Autodesk Inventor part; units mm, degrees
ref_plane "YZ Plane" through (0, 0, 0) normal (1, 0, 0) x (0, 1, 0)
ref_plane "XZ Plane" through (0, 0, 0) normal (0, 1, 0) x (-1, 0, 0)
ref_plane "XY Plane" through (0, 0, 0) normal (0, 0, 1) x (1, 0, 0)
sketch "Sketch1" plane through (0, 0, 0) normal (0, 0, 1) x (1, 0, 0)
  line L0 (-30.48, 28.575) -> (20.32, 28.575)
  line L1 (20.32, 28.575) -> (20.32, -28.575)
  line L2 (20.32, -28.575) -> (-30.48, -28.575)
  line L3 (-30.48, -28.575) -> (-30.48, 28.575)
  line L4 (-25.4, 28.575) -> (25.4, -28.575) construction
  line L5 (25.4, 28.575) -> (-25.4, -28.575) construction
  line L6 (0, 0) -> (0, -19.5531)
  dimension "d0" = 50.8
  dimension "d1" = 57.15
  dimension "d2" = 20.32
  dimension "d3" = 0
extrude "Extrusion1" add sketch "Sketch1" along normal blind 1.27
sketch "Sketch2" plane through (0, 0, 1.27) normal (0, 0, 1) x (1, 0, 0)
  line L0 (-30.48, -28.575) -> (20.32, -28.575)
  line L1 (20.32, -28.575) -> (20.32, 28.575)
  line L2 (20.32, 28.575) -> (-30.48, 28.575)
  line L3 (-30.48, 28.575) -> (-30.48, -28.575)
  line L4 (20.32, 28.575) -> (-30.48, 28.575)
  line L5 (-30.48, -28.575) -> (20.32, -28.575)
  line L6 (20.32, 28.575) -> (-30.48, 28.575)
  line L7 (-30.48, 28.575) -> (-30.48, -28.575)
  line L8 (-30.48, -28.575) -> (20.32, -28.575)
  line L9 (20.32, -28.575) -> (20.32, 28.575)
  line L10 (22.86, 31.115) -> (-30.48, 31.115)
  line L11 (-30.48, -31.115) -> (22.86, -31.115)
  line L12 (22.86, -31.115) -> (22.86, 31.115)
  line L13 (-30.48, 31.115) -> (-30.48, 28.575)
  line L14 (-30.48, 28.575) -> (-30.48, -28.575)
  line L15 (-30.48, -28.575) -> (-30.48, -31.115)
  point P0 (0, 0)
  point P1 (-30.48, 28.575)
  dimension "d6" = 2.54
  dimension "d7" = 2.54
  dimension "d8" = 2.54
extrude "Extrusion2" add sketch "Sketch2" against normal blind 63.5 contours L0 L1 L2 L13 L10 L12 L11 L15
fillet "Fillet1" radius 38.1 2 edges at (-30.48, -29.845, -62.23) (-30.48, 29.845, -62.23)
sketch "Sketch3" plane through (0, 0, 0) normal (0, 0, -1) x (-1, 0, 0)
  line L0 (30.48, -28.575) -> (-20.32, -28.575)
  line L1 (30.48, 28.575) -> (30.48, -28.575)
  line L2 (-20.32, 28.575) -> (30.48, 28.575)
  line L3 (-20.32, -28.575) -> (-20.32, 28.575)
  line L4 (-7.62, -31.115) -> (30.48, -31.115)
  line L5 (30.48, -31.115) -> (30.48, -28.575)
  line L6 (30.48, -28.575) -> (-7.62, -28.575)
  line L7 (-7.62, -28.575) -> (-7.62, -31.115)
  line L8 (30.48, 31.115) -> (-7.62, 31.115)
  line L9 (-7.62, 31.115) -> (-7.62, 28.575)
  line L10 (30.48, 28.575) -> (30.48, 28.575)
  line L11 (30.48, 28.575) -> (30.48, 31.115)
  line L12 (-20.32, 28.575) -> (30.48, 28.575)
  line L13 (30.48, 28.575) -> (30.48, 28.575)
  line L14 (30.48, -28.575) -> (-20.32, -28.575)
  line L15 (26.416, -28.575) -> (23.876, -28.575)
  line L16 (23.876, -28.575) -> (23.876, -26.035)
  line L17 (23.876, -26.035) -> (26.416, -26.035)
  line L18 (26.416, -26.035) -> (26.416, -28.575)
  line L19 (21.336, -28.575) -> (18.796, -28.575)
  line L20 (18.796, -28.575) -> (18.796, -22.225)
  line L21 (18.796, -22.225) -> (21.336, -22.225)
  line L22 (21.336, -22.225) -> (21.336, -28.575)
  line L23 (-20.32, 28.575) -> (30.48, 28.575)
  line L24 (26.416, 28.575) -> (23.876, 28.575)
  line L25 (23.876, 28.575) -> (23.876, 26.035)
  line L26 (23.876, 26.035) -> (26.416, 26.035)
  line L27 (26.416, 26.035) -> (26.416, 28.575)
  line L28 (21.336, 28.575) -> (18.796, 28.575)
  line L29 (18.796, 28.575) -> (18.796, 22.225)
  line L30 (18.796, 22.225) -> (21.336, 22.225)
  line L31 (21.336, 22.225) -> (21.336, 28.575)
  point P0 (0, 0)
  point P1 (30.48, -26.035)
  point P2 (23.876, -28.575)
  point P3 (30.48, 26.035)
  point P4 (23.876, 28.575)
  point P5 (21.336, 28.575)
  point P6 (18.796, 28.575)
  dimension "d12" = 2.54
  dimension "d13" = 2.54
  dimension "d14" = 2.54
  dimension "d15" = 6.35
  dimension "d16" = 2.54
  dimension "d17" = 2.54
  dimension "d18" = 2.54
  dimension "d19" = 2.54
  dimension "d20" = 6.35
  dimension "d21" = 2.54
  dimension "d57" = 6.35
  dimension "d58" = 6.35
  dimension "d59" = 4.064
extrude "Extrusion3" add sketch "Sketch3" along normal blind 25.4 contours L0 L16 L17 L18 | L27 L26 L25 L2 | L0 L20 L21 L22 | L31 L30 L29 L2
sketch "Sketch4" plane through (-30.48, -31.115, 1.27) normal (0, -1, 0) x (1, 0, 0)
  arc A0 (35.54, -42.8168) -> (35.14, -42.4168) centre (35.14, -42.8168) ccw
  line L0 (35.54, -42.8168) -> (35.54, -47.1668)
  line L1 (35.54, -47.1668) -> (37.14, -47.1668)
  line L2 (37.14, -47.1668) -> (37.14, -42.8168)
  arc A1 (37.54, -42.4168) -> (37.14, -42.8168) centre (37.54, -42.8168) ccw
  line L3 (37.54, -42.4168) -> (53.14, -42.4168)
  line L4 (53.14, -42.4168) -> (53.14, -20.3168)
  line L5 (53.14, -20.3168) -> (37.54, -20.3168)
  arc A2 (37.14, -19.9168) -> (37.54, -20.3168) centre (37.54, -19.9168) ccw
  line L6 (37.14, -19.9168) -> (37.14, -15.5668)
  line L7 (37.14, -15.5668) -> (35.54, -15.5668)
  line L8 (35.54, -15.5668) -> (35.54, -19.9168)
  arc A3 (35.14, -20.3168) -> (35.54, -19.9168) centre (35.14, -19.9168) ccw
  line L9 (35.14, -20.3168) -> (31.04, -20.3168)
  line L10 (31.04, -20.3168) -> (31.04, -35.0805)
  spline S0 degree 3 poles (31.04, -35.0805) (31.04, -35.2107) (31.032, -35.3398) (31.0199, -35.4684) (31.0078, -35.597) (30.9913, -35.725) (30.9724, -35.8527) (30.9346, -36.1082) (30.8875, -36.3608) (30.84, -36.6168) knots 0 0 0 0 0.00039 0.00039 0.00039 0.000781 0.000781 0.000781 0.001562 0.001562 0.001562 0.001562
  spline S1 degree 3 poles (30.84, -36.6168) (30.8871, -36.8706) (30.9346, -37.1252) (30.9724, -37.3806) (30.9913, -37.5084) (31.0077, -37.6365) (31.0199, -37.7651) (31.032, -37.8937) (31.04, -38.0228) (31.04, -38.153) knots -0.000015 -0.000015 -0.000015 -0.000015 0.000759 0.000759 0.000759 0.001147 0.001147 0.001147 0.001534 0.001534 0.001534 0.001534
  line L11 (31.04, -38.153) -> (31.04, -42.4168)
  line L12 (31.04, -42.4168) -> (35.14, -42.4168)
  line L13 (37.34, -42.8168) -> (37.34, -47.1668)
  line L14 (37.34, -15.5668) -> (37.34, -19.9168)
  line L15 (37.34, -42.8168) -> (53.34, -42.8168)
  line L16 (53.34, -42.8168) -> (53.34, -47.1668)
  line L17 (53.34, -47.1668) -> (37.34, -47.1668)
  line L18 (37.34, -47.1668) -> (37.34, -42.8168)
  line L19 (37.34, -19.9168) -> (53.34, -19.9168)
  line L20 (53.34, -19.9168) -> (53.34, -15.5668)
  line L21 (53.34, -15.5668) -> (37.34, -15.5668)
  line L22 (37.34, -15.5668) -> (37.34, -19.9168)
  line L23 (53.34, 0) -> (53.34, -63.5)
  point P0 (30.48, -1.27)
  dimension "d33" = 0
  dimension "d34" = 0
extrude "Extrusion4" add sketch "Sketch4" along normal blind 12.7 contours L15 L16 L17 L13 | L19 L14 L21 L20
sketch "Sketch5" plane through (20.32, -28.575, 0) normal (-1, 0, 0) x (0, 0, 1)
  line L0 (0, 0) -> (0, 57.15)
  line L1 (0, 57.15) -> (-62.23, 57.15)
  line L2 (-62.23, 0) -> (-62.23, 57.15)
  line L3 (0, 0) -> (-62.23, 0)
  line L4 (-62.23, 59.69) -> (-62.23, -2.54)
  line L5 (-62.23, 28.575) -> (-2.2668, 28.575)
  line L6 (-31.1958, 28.575) -> (-31.115, 57.15)
  line L7 (-31.115, 57.15) -> (-37.465, 57.15)
  line L8 (0, 57.15) -> (-62.23, 57.15)
  line L9 (-37.465, 57.15) -> (-37.465, 0)
  line L10 (-62.23, 0) -> (-24.13, 0)
  line L11 (-37.465, 32.1945) -> (-31.1958, 35.814)
  line L12 (-31.1958, 35.814) -> (-24.9267, 32.1945)
  line L13 (-24.9267, 32.1945) -> (-24.9267, 24.9555)
  line L14 (-24.9267, 24.9555) -> (-31.1958, 21.336)
  line L15 (-31.1958, 21.336) -> (-37.465, 24.9555)
  line L16 (-37.465, 24.9555) -> (-37.465, 32.1945)
  point P0 (0, 28.575)
  point P1 (-37.465, 28.575)
  point P2 (-37.465, 32.1945)
  point P3 (-37.465, 24.9555)
  dimension "d28" = 57.15
  dimension "d30" = 6.35
  dimension "d67" = 7.239
extrude "Extrusion5" cut sketch "Sketch5" against normal blind 2.54 contours L12 L13 L5 L6 | L6 L5 L9 L11 L12 | L9 L5 L13 L14 L15
sketch "Sketch6" plane through (-30.48, 31.115, 1.27) normal (0, 1, 0) x (1, 0, 0)
  circle A0 centre (29.21, 44.45) radius 2.54
  line L0 (53.34, 0) -> (53.34, 63.5)
  line L1 (53.34, 0) -> (0, 0)
  point P0 (30.48, 1.27)
  dimension "d38" = 5.08
  dimension "d41" = 24.13
  dimension "d42" = 44.45
extrude "Extrusion6" cut sketch "Sketch6" against normal blind 2.54
chamfer "Chamfer3" distance 12.7 angle 25 1 edges at (14.86, -31.115, -45.8968) measured on face at (17.5267, -39.5817, -45.8968)
chamfer "Chamfer4" distance 12.7 angle 25 1 edges at (14.86, -31.115, -14.2968) measured on face at (17.5267, -39.5817, -14.2968)
sketch "Sketch8" plane through (-30.48, -43.815, 1.27) normal (0, -1, 0) x (1, 0, 0)
  line L0 (53.34, -42.8168) -> (37.34, -42.8168)
  line L1 (50.5178, -53.0889) -> (46.99, -53.0889)
  line L2 (46.99, -53.0889) -> (46.99, -42.8168)
  line L3 (46.99, -42.8168) -> (50.5178, -42.8168)
  line L4 (50.5178, -42.8168) -> (50.5178, -53.0889)
  line L5 (37.34, -53.0889) -> (53.34, -53.0889)
  line L6 (53.34, -53.0889) -> (53.34, -47.1668)
  point P0 (30.48, -1.27)
  dimension "d52" = 2.8222
  dimension "d53" = 6.35
extrude "Extrusion7" cut sketch "Sketch8" against normal blind 12.7
sketch "Sketch9" plane through (0, 0, 0) normal (0, 0, -1) x (-1, 0, 0)
  line L0 (18.796, -22.225) -> (21.336, -22.225)
  line L1 (21.336, -22.225) -> (21.336, -28.575)
  line L2 (23.876, -28.575) -> (21.336, -28.575)
  line L3 (23.876, -28.575) -> (23.876, -26.035)
  line L4 (23.876, -26.035) -> (26.416, -26.035)
  line L5 (26.416, -26.035) -> (26.416, -28.575)
  line L6 (30.48, -28.575) -> (26.416, -28.575)
  line L7 (30.48, 28.575) -> (30.48, -28.575)
  line L8 (26.416, 28.575) -> (30.48, 28.575)
  line L9 (26.416, 28.575) -> (26.416, 26.035)
  line L10 (26.416, 26.035) -> (23.876, 26.035)
  line L11 (23.876, 26.035) -> (23.876, 28.575)
  line L12 (21.336, 28.575) -> (23.876, 28.575)
  line L13 (21.336, 28.575) -> (21.336, 22.225)
  line L14 (21.336, 22.225) -> (18.796, 22.225)
  line L15 (-20.32, 28.575) -> (18.796, 28.575)
  line L16 (-20.32, -28.575) -> (-20.32, 28.575)
  line L17 (18.796, -28.575) -> (-20.32, -28.575)
  line L18 (18.796, -28.575) -> (18.796, -22.225)
  line L19 (18.796, 22.225) -> (18.796, 28.575)
  line L20 (-20.32, -28.575) -> (-20.32, 28.575)
  line L21 (21.336, -22.225) -> (-20.32, -22.225)
  line L22 (-20.32, -22.225) -> (-20.32, -19.05)
  line L23 (-20.32, -19.05) -> (21.336, -19.05)
  line L24 (21.336, -19.05) -> (21.336, -22.225)
  line L25 (21.336, 22.225) -> (-20.32, 22.225)
  line L26 (-20.32, 22.225) -> (-20.32, 19.05)
  line L27 (-20.32, 19.05) -> (21.336, 19.05)
  line L28 (21.336, 19.05) -> (21.336, 22.225)
  point P0 (0, 0)
  point P1 (-20.32, -22.225)
  dimension "d56" = 6.35
  dimension "d60" = 3.175
  dimension "d61" = 3.175
extrude "Extrusion8" add sketch "Sketch9" along normal blind 25.4 contours L21 L16 L23 L24 L0 | L16 L25 L14 L28 L27
chamfer "Chamfer5" distance 6.35 angle 45 2 edges at (-18.796, -22.225, -12.7) (-18.796, 22.225, -12.7)
sketch "Sketch10" plane through (-30.48, 31.115, 1.27) normal (0, 1, 0) x (1, 0, 0)
  circle A0 centre (29.21, 44.45) radius 2.54
  arc A1 (38.1, 63.5) -> (0, 25.4) centre (38.1, 25.4) ccw
  line L0 (0, 0) -> (0, 25.4)
  line L1 (53.34, 0) -> (0, 0)
  line L2 (53.34, 0) -> (53.34, 63.5)
  line L3 (38.1, 63.5) -> (53.34, 63.5)
  arc A2 (38.1, 63.5) -> (0, 25.4) centre (38.1, 25.4) ccw
  line L4 (26.67, 61.7451) -> (29.21, 59.2051)
  line L5 (26.67, 61.7451) -> (30.2621, 61.7451) construction
  line L6 (29.21, 59.2051) -> (31.75, 62.9671)
  arc A3 (31.75, 62.9671) -> (26.67, 61.7451) centre (38.1, 25.4) ccw
  point P0 (30.48, 1.27)
  dimension "d68" = 45
extrude "Extrusion9" cut sketch "Sketch10" against normal blind 2.54 contours L6 L4 A1
properties part number "Base_3DPrint"
Here's how the part is built. I have some questions about the finished solid (model axes, mm). A direction names the side the tool comes from. Round coordinates to 2 decimals unless told otherwise and drop trailing zeros. Order: outer loops, then holes, each group sorted by start corner. A loop starts at its lowest first (then second) coordinate and runs counter-clockwise, first axis right, second up. Notation, with made-up numbers: M 15,41.5 L 63,41.5 A21 ccw 63,45.5 Z; hole C 62,78 d4. An arc over 180 degrees is marked long. Answer as CSV lines item,"result".
Item 1: Imagine slicing it at A-A on z = -43.18. List the corners of the cut face in (x, y) for me (3 decimals), and give its area (3 significant figures).
From the geometry:
outline,"M -25.376,-31.115 L 6.86,-31.115 L 6.86,-43.815 L 16.51,-43.815 L 16.51,-31.115 L 20.038,-31.115 L 20.038,-43.815 L 22.86,-43.815 L 22.86,31.115 L 1.27,31.115 L 1.27,28.575 L 20.32,28.575 L 20.32,-28.575 L -25.376,-28.575 Z; M -25.376,28.575 L -3.81,28.575 L -3.81,31.115 L -25.376,31.115 Z"
area,"536 mm2"
Item 2: Please list where these lines run through material, in increasing order: L1, parallel to Y at x = 17, z = -17.5 (3 decimals); L2, parallel to Y at x = 1.5, z = -46 (3 decimals); L3, parallel to Z at x = -1.27, y = 29.8. Write a range as [from, to].
From the geometry:
L1,"[-43.815, -28.575], [-22.225, -19.05], [19.05, 22.225], [28.575, 31.115]"
L2,"[-31.115, -28.575], [28.575, 31.115]"
L3,"[-57.94, -45.72], [-40.64, 1.27]"
Item 3: Imagine slicing it at D-D on z = -33. List the corners of the cut face in (x, y) for me (3 decimals), and give its area (3 significant figures).
From the geometry:
outline,"M -29.433,-31.115 L 22.86,-31.115 L 22.86,-6.197 L 20.32,-6.197 L 20.32,-28.575 L -29.433,-28.575 Z; M -29.433,28.575 L 20.32,28.575 L 20.32,6.197 L 22.86,6.197 L 22.86,31.115 L -29.433,31.115 Z"
area,"379 mm2"
Item 4: Which directions (+Z, -Z, +X, -X, +Y, -Y) give clear straight access to the entire face, cutting with the end or side of a thin tool? Please do faces 1 (the flat face through (4, -22.225, -13)), 2 (the flat face through (-2.558, 29.863, -59.223)), 3 (the flat face through (21.572, -5.455, -34.287)).
From the geometry:
face 1,"-Z"
face 2,"-Z, +Y"
face 3,"+X, -X"
Item 5: Imagine slicing it at C-C on y = 18. List the corners of the cut face in (x, z) for me.
From the geometry:
outline,"M -30.48,0 L 20.32,0 L 20.32,-62.23 L 22.86,-62.23 L 22.86,1.27 L -30.48,1.27 Z"
Item 6: For pin 1 (17 mm diameter, centred on y = -11.5, z = -19.5, fed in from -X); pin 2 (5 mm diameter, centred on y = -36.5, z = -47, fed in from -X); pin 3 (5 mm diameter, centred on y = -10.5, z = -15.5, fed in from -X); pin 4 (8 mm diameter, centred on y = -34.5, z = -12.5, fed in from -X), each with a flat end and sliding along its axis, tell me the tip position at first contact or that it passes through.
From the geometry:
pin 1,"x = -21.34"
pin 2,"x = 6.86"
pin 3,"x = 20.32"
pin 4,"x = -30.48"
Item 7: We'd pull the mould along Z, two halves only. Please class faces 4 (the flat face through (21.572, 5.404, -34.374)), 5 (the flat face through (-23.876, -27, -13)), 6 (the flat face through (-5, -22, -25.4)): +Z half, -Z half, draft (parallel to the pull), parting line (faces both ways), or undercut.
From the geometry:
face 4,"undercut"
face 5,"draft"
face 6,"-Z half"
